Could you check a few things on this model? Use its own coordinates, in mm. Face numbers are marked on the shaded views. A direction names the side the tool comes from. Round coordinates to 2 decimals unless told otherwise and drop trailing zeros. Loops run counter-clockwise (first coordinate to the right, second up) from the corner with the lowest first, then second, coordinate; pieces in that order, holes last. Notation, with made-up numbers: (38.25, -7) -> (59.25, -7) arc R18 cw to (59.25, 17) -> close; hole circle Ø9 at (-24, 13.25). An arc over 180 degrees is marked (long way). One line per item, written item: value.
from build123d import *

# Parameters (mm, degrees)
F0_W      = 5
F0_H      = 9
F0_W_2    = 23
F1_DEPTH  = 3
F2_DEPTH  = 20
F3_DEPTH  = 9
F0_H_2    = 15
F4_DEPTH  = 5
F5_R      = 0.5
F6_DEPTH  = 25
F7_W      = 6.5
F7_H      = 12.5
F7_R      = 0.9
F8_DEPTH  = 2
F9_R      = 0.9
F10_DEPTH = 25
F11_R     = 0.49999


# Not quite as in the source:
# - a fillet or chamfer is up to 0.001 mm smaller than in the source, because OpenCascade refuses the exact size


with BuildPart() as f1:
    # F0 (on Top) → F1 (new body)
    with BuildSketch(Plane.XY):
        with BuildLine():
            Line((-16.5, 4.5), (-25, 4.5))
            ThreePointArc((-25, 4.5), (-26.767766953, 3.767766953), (-27.5, 2))
            Line((-27.5, 2), (-27.5, 1.5))
            Line((-27.5, 1.5), (-19.5, 1.5))
            ThreePointArc((-19.5, 1.5), (-18, 0), (-19.5, -1.5))
            Line((-19.5, -1.5), (-27.5, -1.5))
            Line((-27.5, -1.5), (-27.5, -2))
            ThreePointArc((-27.5, -2), (-26.767766953, -3.767766953), (-25, -4.5))
            Line((-25, -4.5), (-16.5, -4.5))
            Line((-16.5, -4.5), (-16.5, 4.5))
        make_face()
        with BuildLine():
            Line((25, 4.5), (16.5, 4.5))
            Line((16.5, 4.5), (16.5, -4.5))
            Line((16.5, -4.5), (25, -4.5))
            ThreePointArc((25, -4.5), (26.767766953, -3.767766953), (27.5, -2))
            Line((27.5, -2), (27.5, -1.5))
            Line((27.5, -1.5), (19.5, -1.5))
            ThreePointArc((19.5, -1.5), (18, 0), (19.5, 1.5))
            Line((19.5, 1.5), (27.5, 1.5))
            Line((27.5, 1.5), (27.5, 2))
            ThreePointArc((27.5, 2), (26.767766953, 3.767766953), (25, 4.5))
        make_face()
        with Locations((-14, 0)):
            Rectangle(F0_W, F0_H)
        with Locations((14, 0)):
            Rectangle(F0_W, F0_H)
        Rectangle(F0_W_2, F0_H)
    extrude(amount=F1_DEPTH)

    # F0 (on Top) → F2 (join)
    with BuildSketch(Plane.XY):
        with Locations((14, 0)):
            Rectangle(F0_W, F0_H)
        with Locations((-14, 0)):
            Rectangle(F0_W, F0_H)
    extrude(amount=F2_DEPTH)

    # F0 (on Top) → F3 (join)
    with BuildSketch(Plane.XY):
        Rectangle(F0_W_2, F0_H)
    extrude(amount=F3_DEPTH)

    # F0 (on Top) → F4 (join)
    with BuildSketch(Plane.XY):
        with Locations((-14, -12)):
            Rectangle(F0_W, F0_H_2)
    extrude(amount=F4_DEPTH)

    # F5 (on face) → F6 (cut)
    with BuildSketch(Plane.YZ.offset(-11.5)):
        with Locations((-17.5, 2.5)):
            Circle(F5_R)
    extrude(amount=-F6_DEPTH, mode=Mode.SUBTRACT)

    # F7 (on Top) → F8 (join)
    with BuildSketch(Plane.XY):
        with Locations((14.75, -10.75)):
            Rectangle(F7_W, F7_H)
        with Locations((16.5, -14)):
            Circle(F7_R, mode=Mode.SUBTRACT)
        with Locations((16.5, -7.5)):
            Circle(F7_R, mode=Mode.SUBTRACT)
    extrude(amount=F8_DEPTH)

    # F9 (on face) → F10 (cut)
    with BuildSketch(Plane.XZ.offset(4.5)):
        with Locations((-14, 15)):
            Circle(F9_R)
        with Locations((14, 15)):
            Circle(F9_R)
    extrude(amount=-F10_DEPTH, mode=Mode.SUBTRACT)

    # F11 (radius 0.5 in the source; OpenCascade refuses exactly that, so slightly less here)
    f11_edges = [f1.edges().sort_by_distance(p)[0] for p in [
        (11.5, -17, 1),
        (18, -17, 1),
        (-11.5, -19.5, 2.5),
        (-16.5, -19.5, 2.5),
        (-16.5, -4.5, 12.5),
        (11.5, -4.5, 14.5),
        (-11.5, -4.5, 14.5),
        (16.5, -4.5, 11.5),
        (11.5, 4.5, 14.5),
        (-11.5, 4.5, 14.5),
        (-16.5, 4.5, 11.5),
        (16.5, 4.5, 11.5),
        (-27.5, 1.5, 1.5),
        (-27.5, -1.5, 1.5),
        (27.5, 1.5, 1.5),
        (27.5, -1.5, 1.5),
    ]]
    fillet(f11_edges, radius=F11_R)


solid = f1.part
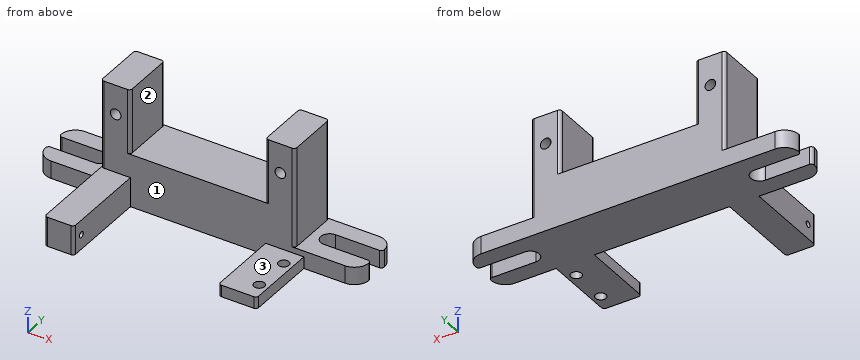
(1) If we section it at B-B, the plane z = 18.25: Please give me the cut outline in (x, y), then the cut area to 3 significant figures.
Recorded:
outline: (-16.5, -4) arc R0.5 ccw to (-16, -4.5) -> (-12, -4.5) arc R0.5 ccw to (-11.5, -4) -> (-11.5, 4) arc R0.5 ccw to (-12, 4.5) -> (-16, 4.5) arc R0.5 ccw to (-16.5, 4) -> close; (11.5, -4) arc R0.5 ccw to (12, -4.5) -> (16, -4.5) arc R0.5 ccw to (16.5, -4) -> (16.5, 4) arc R0.5 ccw to (16, 4.5) -> (12, 4.5) arc R0.5 ccw to (11.5, 4) -> close
area: 89.6 mm²
(2) For the marked faces 1, 2 and 3, which set-ups out of +Z, -Z, +X, -X, +Y, -Y let a thin tool reach every point of the face, with its end or its side?
Recorded:
face 1: +Z, -Y
face 2: +Z, +Y, -Y
face 3: +Z, +X, -Y
(3) I'm going to push flat-ended pins straight in: pin 1 Ø1.6 at (y, z) = (-9.5, 1.5) entering from -X; pin 2 Ø4 at (y, z) = (-14.5, 2) entering from +X; pin 3 Ø6 at (x, y) = (0, -1) entering from +Z. Where does each tip first touch, or does it pass through?
Recorded:
pin 1: x = -16.5
pin 2: x = 18
pin 3: z = 9
(4) If we section it at A-A, the plane x = -14: Please give me the cut outline in (y, z).
Recorded:
outline: (-19.5, 0) -> (4.5, 0) -> (4.5, 14.1) -> (-4.5, 14.1) -> (-4.5, 5) -> (-19.5, 5) -> close; (-4.5, 15.9) -> (4.5, 15.9) -> (4.5, 20) -> (-4.5, 20) -> close; hole circle Ø1 at (-17.5, 2.5)
(5) If I drill on L1, parallel to Y at x = 16.5, z = 0.65; L2, parallel to Z at x = -14, y = -2; L3, parallel to X at y = -1.5, z = 17.25, over which ranges is the centre line in solid material (lowest first)?
Recorded:
L1: -17 to -14.9, -13.1 to -8.4, -6.6 to 4.5
L2: 0 to 14.1, 15.9 to 20
L3: -16.5 to -11.5, 11.5 to 16.5
(6) If we section it at D-D, the plane x = 20.5: Please give me the cut outline in (y, z), then the cut area to 3 significant figures.
Recorded:
outline: (-4.5, 0) -> (-1.5, 0) -> (-1.5, 3) -> (-4.5, 3) -> close; (1.5, 0) -> (4.5, 0) -> (4.5, 3) -> (1.5, 3) -> close
area: 18.0 mm²
(7) If we section it at C-C, the plane y = -9.75: Please give me the cut outline in (x, z).
Recorded:
outline: (-16.5, 0) -> (-11.5, 0) -> (-11.5, 5) -> (-16.5, 5) -> close; (11.5, 0) -> (18, 0) -> (18, 2) -> (11.5, 2) -> close
